CAD build for the part. Positions are in the model's coordinates, mm. Face numbers are marked on the shaded views. A direction names the side the tool comes from. Give positions to 0.01 mm unless a question says otherwise; leave off trailing zeros. Loops run counter-clockwise (first coordinate to the right, second up) from the corner with the lowest first, then second, coordinate; pieces in that order, holes last. Notation, with made-up numbers: (57.5, 61) -> (100.5, 61) arc R10 ccw to (100.5, 70) -> close; hole circle Ø1 at (88, 16). An arc over 180 degrees is marked (long way). Use one line per item in the form item = value.
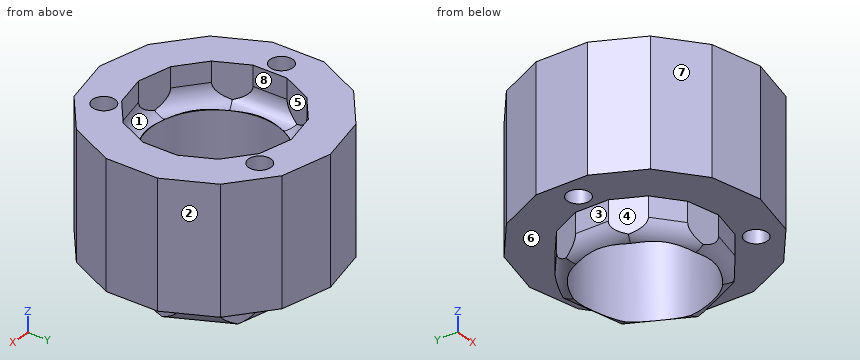
```python
from build123d import *

# Parameters (mm, degrees)
F0_R         = 12.5
F1_DEPTH     = 12.5
F2_R         = 2.25
F3_DEPTH     = 25
F4_R         = 12.5
F5_DEPTH     = 7.5
F6_R         = 12.5
F7_DEPTH     = 7.5
F8_T4_DEPTH  = 24.3016555368
F8_S5_R      = 12.5
F8_T6_DEPTH  = 15
F8_T11_DEPTH = 24.3016555368
F8_S12_R     = 12.5
F8_T13_DEPTH = 14
F8_T17_DEPTH = 24.3016555368
F8_S18_R     = 12.5
F8_T19_DEPTH = 15
F8_T24_DEPTH = 24.3016555368
F8_S25_R     = 12.5
F8_T26_DEPTH = 15
F8_T30_DEPTH = 24.3016555368
F8_S31_R     = 12.5
F8_T32_DEPTH = 15
F8_T37_DEPTH = 24.3016555368
F8_S38_R     = 12.5
F8_T39_DEPTH = 15
F8_T44_DEPTH = 24.3016555368
F8_S45_R     = 12.5
F8_T46_DEPTH = 15
F9_T1_DEPTH  = 24.050587715
F9_T3_DEPTH  = 24.050587715
F9_T5_DEPTH  = 24.050587715
F9_T7_DEPTH  = 24.050587715
F9_T9_DEPTH  = 24.050587715
F9_T11_DEPTH = 24.050587715
F9_T13_DEPTH = 24.050587715


# Not quite as in the source:
# - a fillet or chamfer that OpenCascade refuses, or shapes differently, is made with other operations: its cross-section is extruded or revolved along the edge and cut away or added


with BuildPart() as f1:
    # F0 (on Top) → F1 (new body, symmetric)
    with BuildSketch(Plane.XY):
        Polygon((22.5, -5.1354781738), (22.5, 5.1354781738), (18.0435990556, 14.3892900865), (10.013442028, 20.7931266245), (0, 23.0786294236), (-10.013442028, 20.7931266245), (-18.0435990556, 14.3892900865), (-22.5, 5.1354781738), (-22.5, -5.1354781738), (-18.0435990556, -14.3892900865), (-10.013442028, -20.7931266245), (0, -23.0786294236), (10.013442028, -20.7931266245), (18.0435990556, -14.3892900865), align=None)
        Circle(F0_R, mode=Mode.SUBTRACT)
    extrude(amount=F1_DEPTH, both=True)

    # F2 (on face) → F3 (cut)
    with BuildSketch(Plane.XY.offset(12.5)):
        with Locations((9, 15.5884572681)):
            Circle(F2_R)
        with Locations((-18, 0)):
            Circle(F2_R)
        with Locations((9, -15.5884572681)):
            Circle(F2_R)
    extrude(amount=-F3_DEPTH, mode=Mode.SUBTRACT)

    # F4 (on face) → F5 (cut)
    with BuildSketch(Plane.XY.offset(12.5)):
        Polygon((14.9, -3.4008277684), (14.9, 3.4008277684), (11.9488722635, 9.5289076573), (6.6311238319, 13.7696705203), (0, 15.2831812628), (-6.6311238319, 13.7696705203), (-11.9488722635, 9.5289076573), (-14.9, 3.4008277684), (-14.9, -3.4008277684), (-11.9488722635, -9.5289076573), (-6.6311238319, -13.7696705203), (0, -15.2831812628), (6.6311238319, -13.7696705203), (11.9488722635, -9.5289076573), align=None)
        Circle(F4_R, mode=Mode.SUBTRACT)
    extrude(amount=-F5_DEPTH, mode=Mode.SUBTRACT)

    # F6 (on face) → F7 (join)
    with BuildSketch(Plane(origin=(0, 0, -12.5), x_dir=(1, 0, 0), z_dir=(0, 0, -1))):
        Polygon((14.35, -3.2752938575), (14.35, 3.2752938575), (11.5078065088, 9.1771694552), (6.3863508045, 13.2613940917), (0, 14.719036988), (-6.3863508045, 13.2613940917), (-11.5078065088, 9.1771694552), (-14.35, 3.2752938575), (-14.35, -3.2752938575), (-11.5078065088, -9.1771694552), (-6.3863508045, -13.2613940917), (0, -14.719036988), (6.3863508045, -13.2613940917), (11.5078065088, -9.1771694552), align=None)
        Circle(F6_R, mode=Mode.SUBTRACT)
    extrude(amount=F7_DEPTH)

    # F8: fillet of radius 3.5 on 7 edges, made by hand


with BuildPart() as f8_tool2:
    # F8_s3 → F8_t4 (new body)
    with BuildSketch(Plane(origin=(9.4998996874, 7.5759171977, 0), x_dir=(0, 0, 1), z_dir=(-0.7818314825, -0.6234898019, 0))):
        with BuildLine():
            ThreePointArc((5, 11.4), (6.0251262658, 13.8748737342), (8.5, 14.9))
            Line((8.5, 14.9), (5, 14.9))
            Line((5, 14.9), (5, 11.4))
        make_face()
    extrude(amount=F8_T4_DEPTH)

    # F8_s5 → F8_t6 (cut, symmetric)
    with BuildSketch(Plane.XY.offset(6.8)):
        Circle(F8_S5_R)
    extrude(amount=F8_T6_DEPTH, both=True, mode=Mode.SUBTRACT)

    split(bisect_by=Plane(origin=(-13.4244361317, 6.4648677129, 0), x_dir=(0, 0, 1), z_dir=(0.9009688679, -0.4338837391, 0)), keep=Keep.TOP)


with BuildPart() as f1_1:
    add(f1.part)

    # F8_t1: union F8_tool2
    add(f8_tool2.part)


with BuildPart() as f8_tool9:
    # F8_s10 → F8_t11 (new body)
    with BuildSketch(Plane.XZ.offset(-12.1508277684)):
        with BuildLine():
            ThreePointArc((-11.4, 5), (-13.8748737342, 6.0251262658), (-14.9, 8.5))
            Line((-14.9, 8.5), (-14.9, 5))
            Line((-14.9, 5), (-11.4, 5))
        make_face()
    extrude(amount=F8_T11_DEPTH)

    # F8_s12 → F8_t13 (cut, symmetric)
    with BuildSketch(Plane.XY.offset(6.8)):
        Circle(F8_S12_R)
    extrude(amount=F8_T13_DEPTH, both=True, mode=Mode.SUBTRACT)


with BuildPart() as f1_2:
    add(f1_1.part)

    # F8_t8: union F8_tool9
    add(f8_tool9.part)


with BuildPart() as f8_tool15:
    # F8_s16 → F8_t17 (new body)
    with BuildSketch(Plane(origin=(-9.4998996874, 7.5759171977, 0), x_dir=(0, 0, 1), z_dir=(0.7818314825, -0.6234898019, 0))):
        with BuildLine():
            ThreePointArc((5, 11.4), (6.0251262658, 13.8748737342), (8.5, 14.9))
            Line((8.5, 14.9), (5, 14.9))
            Line((5, 14.9), (5, 11.4))
        make_face()
    extrude(amount=F8_T17_DEPTH)

    # F8_s18 → F8_t19 (cut, symmetric)
    with BuildSketch(Plane.XY.offset(6.8)):
        Circle(F8_S18_R)
    extrude(amount=F8_T19_DEPTH, both=True, mode=Mode.SUBTRACT)

    split(bisect_by=Plane.YZ.offset(-14.9), keep=Keep.TOP)


with BuildPart() as f1_3:
    add(f1_2.part)

    # F8_t14: union F8_tool15
    add(f8_tool15.part)


with BuildPart() as f8_tool22:
    # F8_s23 → F8_t24 (new body)
    with BuildSketch(Plane(origin=(-11.8461811475, -2.7038135434, 0), x_dir=(0, 0, 1), z_dir=(0.9749279122, 0.222520934, 0))):
        with BuildLine():
            ThreePointArc((8.5, 14.9), (6.0251262658, 13.8748737342), (5, 11.4))
            Line((5, 11.4), (5, 14.9))
            Line((5, 14.9), (8.5, 14.9))
        make_face()
    extrude(amount=F8_T24_DEPTH)

    # F8_s25 → F8_t26 (cut, symmetric)
    with BuildSketch(Plane.XY.offset(6.8)):
        Circle(F8_S25_R)
    extrude(amount=F8_T26_DEPTH, both=True, mode=Mode.SUBTRACT)


with BuildPart() as f1_4:
    add(f1_3.part)

    # F8_t21: union F8_tool22
    add(f8_tool22.part)


with BuildPart() as f8_tool28:
    # F8_s29 → F8_t30 (new body)
    with BuildSketch(Plane(origin=(-5.2720465855, -10.9475175386, 0), x_dir=(0, 0, 1), z_dir=(0.4338837391, 0.9009688679, 0))):
        with BuildLine():
            ThreePointArc((5, 11.4), (6.0251262658, 13.8748737342), (8.5, 14.9))
            Line((8.5, 14.9), (5, 14.9))
            Line((5, 14.9), (5, 11.4))
        make_face()
    extrude(amount=F8_T30_DEPTH)

    # F8_s31 → F8_t32 (cut, symmetric)
    with BuildSketch(Plane.XY.offset(6.8)):
        Circle(F8_S31_R)
    extrude(amount=F8_T32_DEPTH, both=True, mode=Mode.SUBTRACT)

    split(bisect_by=Plane(origin=(9.2899980477, -11.6492890888, 0), x_dir=(0, 0, 1), z_dir=(-0.6234898019, 0.7818314825, 0)), keep=Keep.TOP)


with BuildPart() as f1_5:
    add(f1_4.part)

    # F8_t27: union F8_tool28
    add(f8_tool28.part)


with BuildPart() as f8_tool35:
    # F8_s36 → F8_t37 (new body)
    with BuildSketch(Plane(origin=(5.2720465855, -10.9475175386, 0), x_dir=(0, 0, 1), z_dir=(-0.4338837391, 0.9009688679, 0))):
        with BuildLine():
            ThreePointArc((5, 11.4), (6.0251262658, 13.8748737342), (8.5, 14.9))
            Line((8.5, 14.9), (5, 14.9))
            Line((5, 14.9), (5, 11.4))
        make_face()
    extrude(amount=F8_T37_DEPTH)

    # F8_s38 → F8_t39 (cut, symmetric)
    with BuildSketch(Plane.XY.offset(6.8)):
        Circle(F8_S38_R)
    extrude(amount=F8_T39_DEPTH, both=True, mode=Mode.SUBTRACT)

    split(bisect_by=Plane(origin=(9.2899980477, 11.6492890888, 0), x_dir=(0, 0, 1), z_dir=(-0.6234898019, -0.7818314825, 0)), keep=Keep.TOP)


with BuildPart() as f1_6:
    add(f1_5.part)

    # F8_t34: union F8_tool35
    add(f8_tool35.part)


with BuildPart() as f8_tool42:
    # F8_s43 → F8_t44 (new body)
    with BuildSketch(Plane(origin=(11.8461811475, -2.7038135434, 0), x_dir=(0, 0, 1), z_dir=(-0.9749279122, 0.222520934, 0))):
        with BuildLine():
            ThreePointArc((5, 11.4), (6.0251262658, 13.8748737342), (8.5, 14.9))
            Line((8.5, 14.9), (5, 14.9))
            Line((5, 14.9), (5, 11.4))
        make_face()
    extrude(amount=F8_T44_DEPTH)

    # F8_s45 → F8_t46 (cut, symmetric)
    with BuildSketch(Plane.XY.offset(6.8)):
        Circle(F8_S45_R)
    extrude(amount=F8_T46_DEPTH, both=True, mode=Mode.SUBTRACT)


with BuildPart() as f1_7:
    add(f1_6.part)

    # F8_t41: union F8_tool42
    add(f8_tool42.part)

    # F9: fillet of radius 3.5 on 7 edges, made by hand

    # F9_s2 → F9_t1 (cut)
    with BuildSketch(Plane(origin=(-5.2175794629, 10.834415393, 0), x_dir=(0, 0, 1), z_dir=(0.4338837391, -0.9009688679, 0))):
        with BuildLine():
            ThreePointArc((-16.5, -14.35), (-18.9748737342, -13.3248737342), (-20, -10.85))
            Line((-20, -10.85), (-20, -14.35))
            Line((-20, -14.35), (-16.5, -14.35))
        make_face()
    extrude(amount=F9_T1_DEPTH, mode=Mode.SUBTRACT)

    # F9_s4 → F9_t3 (cut)
    with BuildSketch(Plane(origin=(-11.7237946339, 2.6758796203, 0), x_dir=(0, 0, 1), z_dir=(0.9749279122, -0.222520934, 0))):
        with BuildLine():
            ThreePointArc((-16.5, -14.35), (-18.9748737342, -13.3248737342), (-20, -10.85))
            Line((-20, -10.85), (-20, -14.35))
            Line((-20, -14.35), (-16.5, -14.35))
        make_face()
    extrude(amount=F9_T3_DEPTH, mode=Mode.SUBTRACT)

    # F9_s6 → F9_t5 (cut)
    with BuildSketch(Plane(origin=(-9.4017533237, -7.4976480845, 0), x_dir=(0, 0, 1), z_dir=(0.7818314825, 0.6234898019, 0))):
        with BuildLine():
            ThreePointArc((-16.5, -14.35), (-18.9748737342, -13.3248737342), (-20, -10.85))
            Line((-20, -10.85), (-20, -14.35))
            Line((-20, -14.35), (-16.5, -14.35))
        make_face()
    extrude(amount=F9_T5_DEPTH, mode=Mode.SUBTRACT)

    # F9_s8 → F9_t7 (cut)
    with BuildSketch(Plane.XZ.offset(-12.0252938575)):
        with BuildLine():
            ThreePointArc((-14.35, -16.5), (-13.3248737342, -18.9748737342), (-10.85, -20))
            Line((-10.85, -20), (-14.35, -20))
            Line((-14.35, -20), (-14.35, -16.5))
        make_face()
    extrude(amount=F9_T7_DEPTH, mode=Mode.SUBTRACT)

    # F9_s10 → F9_t9 (cut)
    with BuildSketch(Plane(origin=(9.4017533237, -7.4976480845, 0), x_dir=(0, 0, 1), z_dir=(-0.7818314825, 0.6234898019, 0))):
        with BuildLine():
            ThreePointArc((-16.5, -14.35), (-18.9748737342, -13.3248737342), (-20, -10.85))
            Line((-20, -10.85), (-20, -14.35))
            Line((-20, -14.35), (-16.5, -14.35))
        make_face()
    extrude(amount=F9_T9_DEPTH, mode=Mode.SUBTRACT)

    # F9_s12 → F9_t11 (cut)
    with BuildSketch(Plane(origin=(11.7237946339, 2.6758796203, 0), x_dir=(0, 0, 1), z_dir=(-0.9749279122, -0.222520934, 0))):
        with BuildLine():
            ThreePointArc((-16.5, -14.35), (-18.9748737342, -13.3248737342), (-20, -10.85))
            Line((-20, -10.85), (-20, -14.35))
            Line((-20, -14.35), (-16.5, -14.35))
        make_face()
    extrude(amount=F9_T11_DEPTH, mode=Mode.SUBTRACT)

    # F9_s14 → F9_t13 (cut)
    with BuildSketch(Plane(origin=(5.2175794629, 10.834415393, 0), x_dir=(0, 0, 1), z_dir=(-0.4338837391, -0.9009688679, 0))):
        with BuildLine():
            ThreePointArc((-16.5, -14.35), (-18.9748737342, -13.3248737342), (-20, -10.85))
            Line((-20, -10.85), (-20, -14.35))
            Line((-20, -14.35), (-16.5, -14.35))
        make_face()
    extrude(amount=F9_T13_DEPTH, mode=Mode.SUBTRACT)


solid = f1_7.part
```
1. Cut at B-B, the plane z = -0.5. Write the cut outline in (x, y).
Result sheet:
outline = (-22.5, -5.14) -> (-18.04, -14.39) -> (-10.01, -20.79) -> (0, -23.08) -> (10.01, -20.79) -> (18.04, -14.39) -> (22.5, -5.14) -> (22.5, 5.14) -> (18.04, 14.39) -> (10.01, 20.79) -> (0, 23.08) -> (-10.01, 20.79) -> (-18.04, 14.39) -> (-22.5, 5.14) -> close; hole circle Ø4.5 at (-18, 0); hole circle Ø25 at (0, 0); hole circle Ø4.5 at (9, -15.59); hole circle Ø4.5 at (9, 15.59)
2. Drill centre lines: line 1 (Y direction, x = 9, z = 6.25); line 2 (Y direction, x = 0, z = -1.5); line 3 (Y direction, x = 9, z = -2.5). Where is each one in solid material? Low to high.
Result sheet:
line_1 = -21.02 to -17.84, -13.34 to -11.88, 11.88 to 13.34, 17.84 to 21.02
line_2 = -23.08 to -12.5, 12.5 to 23.08
line_3 = -21.02 to -17.84, -13.34 to -8.67, 8.67 to 13.34, 17.84 to 21.02
3. Tool access for the marked faces 1, 2, 3 and 4: list every direction of +Z, -Z, +X, -X, +Y, -Y with a clear straight run to the whole face (end or side of a thin tool).
Result sheet:
face_1 = +Z
face_2 = +Z, -Z, +X, +Y
face_3 = -Z, -X, +Y, -Y
face_4 = -Z, -X, -Y
4. Mould opens along Y. For the marked faces 5, 6, 7 and 8 say: pulls with the +Y half, pulls with the -Y half, needs draft (parallel to the pull), parting line crosses it, or undercut.
Result sheet:
face_5 = undercut
face_6 = needs draft
face_7 = pulls with the -Y half
face_8 = undercut
5. Drop flat-ended pins along their axis: P1, Ø4, axis at x = 13.5, y = 4.5, coming from the -Z side; P2, Ø1.2, axis at y = 1.5, z = -13.5, coming from the -X side; P3, Ø3, axis at y = 18, z = -2, coming from the -X side. Give the stop position or say it passes through.
Result sheet:
P1 = -19.71
P2 = -14.35
P3 = -15.4
6. Cut at A-A, the plane z = -15. Write the cut outline in (x, y).
Result sheet:
outline = (-14.35, -3.28) -> (-11.51, -9.18) -> (-6.39, -13.26) -> (0, -14.72) -> (6.39, -13.26) -> (11.51, -9.18) -> (14.35, -3.28) -> (14.35, 3.28) -> (11.51, 9.18) -> (6.39, 13.26) -> (0, 14.72) -> (-6.39, 13.26) -> (-11.51, 9.18) -> (-14.35, 3.28) -> close; hole circle Ø25 at (0, 0)
7. Cut at C-C, the plane y = 20. Write the cut outline in (x, z), then the cut area to 3 significant figures.
Result sheet:
outline = (-11.01, -12.5) -> (11.01, -12.5) -> (11.01, 12.5) -> (-11.01, 12.5) -> close
area = 550 mm^2
